Source: CAD feature listing. Evaluate the final solid. Frame: model axes, mm. A direction names the side the tool comes from. Give positions to 0.01 mm unless a question says otherwise; leave off trailing zeros. Loops run counter-clockwise (first coordinate to the right, second up) from the corner with the lowest first, then second, coordinate; pieces in that order, holes last. Notation, with made-up numbers: M 73,76 L 113,76 A26 cw 113,104 Z; hole C -14.5,33 d11. An arc over 180 degrees is marked long. Put each result on its own line as item: value.
from build123d import *

# Parameters (mm, degrees)
EXTRUDE_1_DEPTH          = 8
EXTRUDE_2_DEPTH          = 1
CUT_EXTRUDE_1_DEPTH      = 43.00279577
CUT_EXTRUDE_1_DEPTH_BACK = 43.00279577


with BuildPart() as part:
    # Эскиз1 → Бобышка-Вытянуть1 (new body)
    with BuildSketch(Plane(origin=(0, 0, 0), x_dir=(0, 0, -1), z_dir=(1, 0, 0))):
        with BuildLine():
            Line((-30.474082362, -9.45), (30.474082362, -9.45))
            ThreePointArc((30.474082362, -9.45), (39.924082362, 0), (30.474082362, 9.45))
            Line((30.474082362, 9.45), (-30.474082362, 9.45))
            ThreePointArc((-30.474082362, 9.45), (-39.924082362, 0), (-30.474082362, -9.45))
        make_face()
        with BuildLine():
            Line((-30.474082362, -7.95), (30.474082362, -7.95))
            ThreePointArc((30.474082362, -7.95), (38.424082362, 0), (30.474082362, 7.95))
            Line((30.474082362, 7.95), (-30.474082362, 7.95))
            ThreePointArc((-30.474082362, 7.95), (-38.424082362, 0), (-30.474082362, -7.95))
        make_face(mode=Mode.SUBTRACT)
    extrude(amount=EXTRUDE_1_DEPTH)

    # Эскиз2 → Бобышка-Вытянуть2 (add)
    with BuildSketch(Plane(origin=(8, 0, 0), x_dir=(0, 0, -1), z_dir=(1, 0, 0))):
        with BuildLine():
            Line((-30.474082362, -9.45), (30.474082362, -9.45))
            ThreePointArc((30.474082362, -9.45), (39.924082362, 0), (30.474082362, 9.45))
            Line((30.474082362, 9.45), (-30.474082362, 9.45))
            ThreePointArc((-30.474082362, 9.45), (-39.924082362, 0), (-30.474082362, -9.45))
        make_face()
    extrude(amount=EXTRUDE_2_DEPTH)

    # Эскиз3 → Вырез-Вытянуть1 (cut, two sides: drawn at the far end of the back side and taken through both)
    with BuildSketch(Plane(origin=(9, 0, 0), x_dir=(0, 0, -1), z_dir=(1, 0, 0)).offset(-CUT_EXTRUDE_1_DEPTH_BACK)):
        Polygon((-30.474082362, 9.45), (-30.474082362, -9.45), (-59.348186325, -9.45), (-44.911134344, 15.375653675), align=None)
    extrude(amount=CUT_EXTRUDE_1_DEPTH + CUT_EXTRUDE_1_DEPTH_BACK, mode=Mode.SUBTRACT)


solid = part.part
1. Section query B-B (y = 0). Output: boundary loops of the cut face in (x, z), plus the area to 3 significant figures.
Found:
outline: M 0,-39.92 L 9,-39.92 L 9,30.47 L 8,30.47 L 8,-38.42 L 0,-38.42 Z
area: 82.4 mm^2
2. Material intervals for line 1 (Y direction, x = 5, z = 18.5); line 2 (X direction, y = 5, z = 6); line 3 (Y direction, x = 3, z = -35.5), sorted ascending. Write a range as from..to.
Found:
line 1: -9.45..-7.95, 7.95..9.45
line 2: 8..9
line 3: -8..-6.16, 6.16..8
3. Access query for faces 1 (the cylindrical face through (3.944, -0.175, -38.422)), 2 (the flat face through (4, 9.45, 0)). Directions: +Z, -Z, +X, -X, +Y, -Y. A direction counts if a zero-diameter tool reaches every point of the face in a straight line with its end or side. Return the directions, or none.
Found:
face 1: +Z, -X
face 2: +Z, -Z, +X, -X, +Y
4. Draft query along Y for faces 3 (the flat face through (4, -9.45, 0)), 4 (the flat face through (8.15, -0.66, 30.474)), 5 (the flat face through (4, 7.95, 0)), 6 (the flat face through (4, -7.95, 0)). Return one class per face: pulls with the +Y half, pulls with the -Y half, needs draft (parallel to the pull), parting line crosses it, or undercut.
Found:
face 3: pulls with the -Y half
face 4: needs draft
face 5: undercut
face 6: undercut
5. Section query C-C (z = 1). Output: boundary loops of the cut face in (x, y).
Found:
outline: M 0,-9.45 L 9,-9.45 L 9,9.45 L 0,9.45 L 0,7.95 L 8,7.95 L 8,-7.95 L 0,-7.95 Z
6. Section query D-D (y = 5.25). Output: boundary loops of the cut face in (x, z), plus the area to 3 significant figures.
Found:
outline: M 0,-38.33 L 9,-38.33 L 9,30.47 L 8,30.47 L 8,-36.44 L 0,-36.44 Z
area: 83.9 mm^2
7. Section query A-A (x = 3.75). Output: boundary loops of the cut face in (y, z), plus the area to 3 significant figures.
Found:
outline: M -9.45,-30.47 A9.45 ccw 9.45,-30.47 L 9.45,30.47 L 7.95,30.47 L 7.95,-30.47 A7.95 cw -7.95,-30.47 L -7.95,30.47 L -9.45,30.47 Z
area: 224 mm^2
8. Contact query for flat-ended pins moving along their axis: P1, Ø2, axis at y = -1.5, z = 21, coming from the -X side; P2, Ø3, axis at x = 7.5, y = -3, coming from the +Z side; P3, Ø2, axis at x = 6.5, y = -6.5, coming from the -Z side; P4, Ø2, axis at x = 3, y = -3, coming from the +Z side. Output: stop coordinate, or through.
Found:
P1: x = 8
P2: z = 30.47
P3: z = -38.16
P4: z = -37.34
